Verification items for the finished model (mm, model axes). Give positions to 0.01 mm unless a question says otherwise; leave off trailing zeros. Write each loop counter-clockwise with the first axis right and the second up, starting at its lowest first coordinate (ties: lowest second). Pieces come first, ordered by that corner, then holes. Notation, with made-up numbers: (63.5, 24.25) -> (72.5, 24.25) arc R25 cw to (72.5, 40.25) -> close; hole circle Ø2 at (54.25, -36). An arc over 180 degrees is marked (long way). Answer as CSV lines item,"result". Start each with the question number.
1) Gauge pin test, flat ends, axial feed: pin 1 Ø5.5 at (x, y) = (-34.925, 95.25) entering from -Z; pin 2 Ø0.8 at (x, z) = (-34, 0.5) entering from -Y; pin 3 Ø4 at (x, y) = (-0.11, 12.27) entering from +Z. Record the tip position at first contact, or that the pin passes through.
2) Mould release check, pull along X, two halves, no side actions. Record for faces 1 (the flat face through (-7.453, 80.079, 0.783)), 2 (the cylindrical face through (0.86, 26.83, 0.78)), 3 (the cylindrical face through (-37.671, 100.975, 0.783)): released by +X, released by -X, zero draft, split by the parting line, or undercut.
3) Sectioned sample at D-D on y = 74.5. Record the cut outline in (x, z) (1 decimal), and give its area (3 significant figures).
4) Sectioned sample at B-B on z = 1.2. Give the number of separate pieces and of enclosed holes in the cut face, and give its area (3 significant figures).
5) Sectioned sample at A-A on y = 0. Record the cut outline in (x, z).
6) Sectioned sample at C-C on x = -23.5. Record the cut outline in (y, z).
7) Material ranges on L1, parallel to Y at x = 1, z = 0.9; L2, parallel to Y at x = 1.5, z = 0.95; L3, parallel to X at y = 29.5, z = 0.55, recorded low to high.
Autodesk Inventor part; units mm, degrees
ref_plane "YZ Plane" through (0, 0, 0) normal (1, 0, 0) x (0, 1, 0)
ref_plane "XZ Plane" through (0, 0, 0) normal (0, 1, 0) x (-1, 0, 0)
ref_plane "XY Plane" through (0, 0, 0) normal (0, 0, 1) x (1, 0, 0)
sketch "main" plane through (0, 0, 0) normal (0, 0, 1) x (1, 0, 0)
  arc A0 (-13.083, -30.8821) -> (-6.3594, -42.088) centre (-0.383, -30.8821) ccw
  line L0 (-13.083, -6.7521) -> (-13.083, -30.8821)
  arc A1 (-13.083, -6.7521) -> (-19.433, -0.4021) centre (-19.433, -6.7521) ccw
  line L1 (-6.3594, -42.088) -> (9.3288, -50.4551)
  line L2 (29.7795, 10.9635) -> (29.7795, -38.5021)
  arc A2 (29.7795, 10.9635) -> (27.5605, 15.7861) centre (23.4295, 10.9635) ccw
  circle A3 centre (12.317, -44.8521) radius 2.0955
  arc A4 (9.3288, -50.4551) -> (12.317, -51.2021) centre (12.2103, -45.2792) ccw
  line L3 (17.0795, -51.2021) -> (12.317, -51.2021)
  arc A5 (17.0795, -51.2021) -> (29.7795, -38.5021) centre (17.0795, -38.5021) ccw
  circle A6 centre (-22.608, 50.3979) radius 2.0955
  arc A7 (-18.477, 55.2205) -> (-28.958, 50.3979) centre (-22.608, 50.3979) ccw
  line L4 (27.5605, 15.7861) -> (-18.477, 55.2205)
  line L5 (-22.608, -0.4021) -> (-19.433, -0.4021)
  arc A8 (-28.958, 5.9479) -> (-22.608, -0.4021) centre (-22.608, 5.9479) ccw
  line L6 (-28.958, 50.3979) -> (-28.958, 5.9479)
  point P0 (-1.5201, -8.3134)
  dimension "d1" = 4.191
  dimension "d2" = 12.7
  dimension "d3" = 4.191
  dimension "d4" = 12.7
  dimension "d5" = 12.7
  dimension "d6" = 6.35
  dimension "d7" = 6.35
sketch "Sketch1" plane through (0, 0, 0) normal (0, 0, 1) x (1, 0, 0)
  circle A0 centre (-0.1068, 24.9729) radius 2.0955
  circle A1 centre (-0.1068, 12.2729) radius 2.0955
  arc A2 (-25.4, 13.97) -> (-18.6765, 2.7641) centre (-12.7, 13.97) ccw
  line L0 (-25.4, 38.1) -> (-25.4, 13.97)
  arc A3 (-25.4, 38.1) -> (-31.75, 44.45) centre (-31.75, 38.1) ccw
  line L1 (-18.6765, 2.7641) -> (-2.9882, -5.6029)
  line L2 (17.4625, 55.8156) -> (17.4625, 6.35)
  arc A4 (17.4625, 55.8156) -> (15.2434, 60.6383) centre (11.1125, 55.8156) ccw
  circle A5 centre (0, 0) radius 2.0955
  arc A6 (-2.9882, -5.6029) -> (0, -6.35) centre (-0.1068, -0.4271) ccw
  line L3 (4.7625, -6.35) -> (0, -6.35)
  arc A7 (4.7625, -6.35) -> (17.4625, 6.35) centre (4.7625, 6.35) ccw
  circle A8 centre (-34.925, 95.25) radius 2.0955
  arc A9 (-30.7941, 100.0726) -> (-41.275, 95.25) centre (-34.925, 95.25) ccw
  line L4 (15.2434, 60.6383) -> (-30.7941, 100.0726)
  line L5 (-34.925, 44.45) -> (-31.75, 44.45)
  arc A10 (-41.275, 50.8) -> (-34.925, 44.45) centre (-34.925, 50.8) ccw
  line L6 (-41.275, 95.25) -> (-41.275, 50.8)
  dimension "d11" = 4.191
  dimension "d12" = 4.191
extrude "Extrusion1" add sketch "Sketch1" along normal blind 1.5875
properties part number "back_sled" material "Acetal Resin, White"
Ans:
1,pin 1,"stops at z = 0"
1,pin 2,"stops at y = 44.45"
1,pin 3,"passes through"
2,face 1,"released by +X"
2,face 2,"undercut"
2,face 3,"split by the parting line"
3,outline,"(-41.3, 0) -> (-0.9, 0) -> (-0.9, 1.6) -> (-41.3, 1.6) -> close"
3,area,"64.0 mm²"
4,separate pieces,"1"
4,enclosed holes,"4"
4,area,"4,200 mm²"
5,outline,"(-13.49, 0) -> (-2.1, 0) -> (-2.1, 1.59) -> (-13.49, 1.59) -> close; (2.1, 0) -> (15.76, 0) -> (15.76, 1.59) -> (2.1, 1.59) -> close"
6,outline,"(7.29, 0) -> (93.82, 0) -> (93.82, 1.59) -> (7.29, 1.59) -> close"
7,L1,"y = -6.35 to -1.84, 1.84 to 10.49, 14.05 to 23.19, 26.75 to 72.84"
7,L2,"y = -6.35 to -1.46, 1.46 to 10.93, 13.62 to 23.63, 26.32 to 72.41"
7,L3,"x = -25.4 to 17.46"
